Verification items for the finished model (mm, model axes). A direction names the side the tool comes from. Give positions to 0.01 mm unless a question says otherwise; leave off trailing zeros. Put each result on its own line as item: value. Start each with the question number.
from build123d import *

# Parameters (mm, degrees)
SKETCH_1_W             = 23.5
SKETCH_1_H             = 12
EXTRUDE_1_DEPTH        = 571
HOLE_WIZARD_M6_1_D     = 5
HOLE_WIZARD_M6_1_DEPTH = 15
HOLE_WIZARD_M6_1_TIP   = 1.502151548
HOLE_WIZARD_M6_2_D     = 5
HOLE_WIZARD_M6_2_DEPTH = 15
HOLE_WIZARD_M6_2_TIP   = 1.502151548
HOLE_WIZARD_M4_1_D     = 3.3
HOLE_WIZARD_M4_1_DEPTH = 10.1
HOLE_WIZARD_M4_1_TIP   = 0.991420021
HOLE_WIZARD_M6_3_D     = 5
HOLE_WIZARD_M6_3_DEPTH = 15
HOLE_WIZARD_M6_3_TIP   = 1.502151548


with BuildPart() as part:
    # 草图1 → 凸台-拉伸1 (new, symmetric)
    with BuildSketch(Plane(origin=(0, 0, 0), x_dir=(0, 0, -1), z_dir=(1, 0, 0))):
        with BuildLine():
            Line((-14, 15), (-11.5, 15))
            Line((-11.5, 15), (-11.5, 13.5))
            Line((-11.5, 13.5), (-11.4, 13.5))
            ThreePointArc((-11.4, 13.5), (-11.117157288, 13.382842712), (-11, 13.1))
            Line((-11, 13.1), (-11, 12))
            Line((-11, 12), (-9.5, 12))
            Line((-9.5, 12), (-9.5, 15))
            Line((-9.5, 15), (-8, 15))
            Line((-8, 15), (-8, 12.5))
            Line((-8, 12.5), (-5, 12.5))
            Line((-5, 12.5), (-5, 15))
            Line((-5, 15), (5, 15))
            Line((5, 15), (5, 12.5))
            Line((5, 12.5), (8, 12.5))
            Line((8, 12.5), (8, 15))
            Line((8, 15), (9.5, 15))
            Line((9.5, 15), (9.5, 12))
            Line((9.5, 12), (11, 12))
            Line((11, 12), (11, 13.1))
            ThreePointArc((11, 13.1), (11.117157288, 13.382842712), (11.4, 13.5))
            Line((11.4, 13.5), (11.5, 13.5))
            Line((11.5, 13.5), (11.5, 15))
            Line((11.5, 15), (14, 15))
            ThreePointArc((14, 15), (14.707106781, 14.707106781), (15, 14))
            Line((15, 14), (15, 8))
            Line((15, 8), (12.5, 8))
            Line((12.5, 8), (12.5, 5))
            Line((12.5, 5), (15, 5))
            Line((15, 5), (15, -5))
            Line((15, -5), (12.5, -5))
            Line((12.5, -5), (12.5, -8))
            Line((12.5, -8), (15, -8))
            Line((15, -8), (15, -14))
            ThreePointArc((15, -14), (14.707106781, -14.707106781), (14, -15))
            Line((14, -15), (11.5, -15))
            Line((11.5, -15), (11.5, -13.5))
            Line((11.5, -13.5), (11.4, -13.5))
            ThreePointArc((11.4, -13.5), (11.117157288, -13.382842712), (11, -13.1))
            Line((11, -13.1), (11, -12))
            Line((11, -12), (9.5, -12))
            Line((9.5, -12), (9.5, -15))
            Line((9.5, -15), (8, -15))
            Line((8, -15), (8, -12.5))
            Line((8, -12.5), (5, -12.5))
            Line((5, -12.5), (5, -15))
            Line((5, -15), (-5, -15))
            Line((-5, -15), (-5, -12.5))
            Line((-5, -12.5), (-8, -12.5))
            Line((-8, -12.5), (-8, -15))
            Line((-8, -15), (-9.5, -15))
            Line((-9.5, -15), (-9.5, -12))
            Line((-9.5, -12), (-11, -12))
            Line((-11, -12), (-11, -13.1))
            ThreePointArc((-11, -13.1), (-11.117157288, -13.382842712), (-11.4, -13.5))
            Line((-11.4, -13.5), (-11.5, -13.5))
            Line((-11.5, -13.5), (-11.5, -15))
            Line((-11.5, -15), (-14, -15))
            ThreePointArc((-14, -15), (-14.707106781, -14.707106781), (-15, -14))
            Line((-15, -14), (-15, 14))
            ThreePointArc((-15, 14), (-14.707106781, 14.707106781), (-14, 15))
        make_face()
        with BuildLine():
            Line((12, -10.5), (12, -8.5))
            ThreePointArc((12, -8.5), (11.853553391, -8.146446609), (11.5, -8))
            Line((11.5, -8), (-11.5, -8))
            ThreePointArc((-11.5, -8), (-11.853553391, -8.146446609), (-12, -8.5))
            Line((-12, -8.5), (-12, -10.5))
            ThreePointArc((-12, -10.5), (-11.853553391, -10.853553391), (-11.5, -11))
            Line((-11.5, -11), (11.5, -11))
            ThreePointArc((11.5, -11), (11.853553391, -10.853553391), (12, -10.5))
        make_face(mode=Mode.SUBTRACT)
        with BuildLine():
            Line((-11.5, 11), (11.5, 11))
            ThreePointArc((11.5, 11), (11.853553391, 10.853553391), (12, 10.5))
            Line((12, 10.5), (12, 8.5))
            ThreePointArc((12, 8.5), (11.853553391, 8.146446609), (11.5, 8))
            Line((11.5, 8), (-11.5, 8))
            ThreePointArc((-11.5, 8), (-11.853553391, 8.146446609), (-12, 8.5))
            Line((-12, 8.5), (-12, 10.5))
            ThreePointArc((-12, 10.5), (-11.853553391, 10.853553391), (-11.5, 11))
        make_face(mode=Mode.SUBTRACT)
        Rectangle(SKETCH_1_W, SKETCH_1_H, mode=Mode.SUBTRACT)
    extrude(amount=EXTRUDE_1_DEPTH, both=True)

    # M6 螺纹孔1
    with Locations(Plane.XZ.offset(15)):
        with Locations((551, 0), (536, 0), (-536, 0), (-551, 0)):
            Hole(HOLE_WIZARD_M6_1_D / 2, depth=HOLE_WIZARD_M6_1_DEPTH)
            with Locations((0, 0, -(HOLE_WIZARD_M6_1_DEPTH + HOLE_WIZARD_M6_1_TIP / 2))):  # 118° drill point
                Cone(0, HOLE_WIZARD_M6_1_D / 2, HOLE_WIZARD_M6_1_TIP, mode=Mode.SUBTRACT)

    # M6 螺纹孔2
    with Locations(Plane(origin=(0, 15, 0), x_dir=(-1, 0, 0), z_dir=(0, 1, 0))):
        with Locations((551, 0), (536, 0), (-151, 0), (-136, 0), (-221, 0), (-236, 0), (-536, 0), (-551, 0)):
            Hole(HOLE_WIZARD_M6_2_D / 2, depth=HOLE_WIZARD_M6_2_DEPTH)
            with Locations((0, 0, -(HOLE_WIZARD_M6_2_DEPTH + HOLE_WIZARD_M6_2_TIP / 2))):  # 118° drill point
                Cone(0, HOLE_WIZARD_M6_2_D / 2, HOLE_WIZARD_M6_2_TIP, mode=Mode.SUBTRACT)

    # M4 螺纹孔1
    with Locations(Plane.XZ.offset(15)):
        with Locations((479, 0), (319, 0), (159, 0), (-1, 0), (-161, 0), (-321, 0), (-481, 0)):
            Hole(HOLE_WIZARD_M4_1_D / 2, depth=HOLE_WIZARD_M4_1_DEPTH)
            with Locations((0, 0, -(HOLE_WIZARD_M4_1_DEPTH + HOLE_WIZARD_M4_1_TIP / 2))):  # 118° drill point
                Cone(0, HOLE_WIZARD_M4_1_D / 2, HOLE_WIZARD_M4_1_TIP, mode=Mode.SUBTRACT)

    # M6 螺纹孔3
    with Locations(Plane(origin=(0, 0, -15), x_dir=(-1, 0, 0), z_dir=(0, 0, -1))):
        with Locations((-293.5, 0), (-218.5, 0)):
            Hole(HOLE_WIZARD_M6_3_D / 2, depth=HOLE_WIZARD_M6_3_DEPTH)
            with Locations((0, 0, -(HOLE_WIZARD_M6_3_DEPTH + HOLE_WIZARD_M6_3_TIP / 2))):  # 118° drill point
                Cone(0, HOLE_WIZARD_M6_3_D / 2, HOLE_WIZARD_M6_3_TIP, mode=Mode.SUBTRACT)


solid = part.part
Q1. Scan lines: L1, parallel to Y at x = 342, z = -4.75; L2, parallel to Y at x = 259, z = 10; L3, parallel to Z at x = 151, y = 13.45. Record each from-to range of solid material in increasing order.
Q2. Release check for a two-part mould opening along Z. For faces 1 (the face through (8, 6, 0)), 2 (the face through (571, 7, 0)), 3 (the face through (8, 0, 15)) record: pulls with the +Z half, pulls with the -Z half, needs draft (parallel to the pull), parting line crosses it, or undercut.
Q3. Go/stop test with flat-tipped pins: pin 1 (10 mm diameter, centred on x = 355.5, z = -11, fed in from +Y); pin 2 (0.8 mm diameter, centred on x = 30.5, z = -10, fed in from +Y); pin 3 (1.5 mm diameter, centred on x = 247.5, z = -6, fed in from -Y); pin 4 (2 mm diameter, centred on y = -1.5, z = -9.5, fed in from +X). Record where each tip stops, or that it passes through.
Q4. Cross-section at A-A, the plane x = -57. State how many separate pieces and enclosed holes the cut face has, then the cut area to 3 significant figures.
Q5. Set-up check for faces 4 (the face through (-571, 7, 0)), 5 (the face through (8, 11, 0)): record each of +Z, -Z, +X, -X, +Y, -Y from which the full face is reachable in a straight line by a thin tool's end or side.
Ans:
1. L1: y = -15 to -11, -8 to -6, 6 to 8, 11 to 15
1. L2: y = -12 to -11, -8 to -6, 6 to 8, 11 to 12
1. L3: z = -15 to -11.21, -9.5 to -8, -5 to -2.5, 2.5 to 5, 8 to 9.5, 11.21 to 15
2. face 1: undercut
2. face 2: needs draft
2. face 3: pulls with the +Z half
3. pin 1: stops at y = 15
3. pin 2: stops at y = 12
3. pin 3: stops at y = -12.5
3. pin 4: passes through
4. separate pieces: 1
4. enclosed holes: 3
4. area: 407 mm^2
5. face 4: +Z, -Z, -X, +Y, -Y
5. face 5: +X, -X
